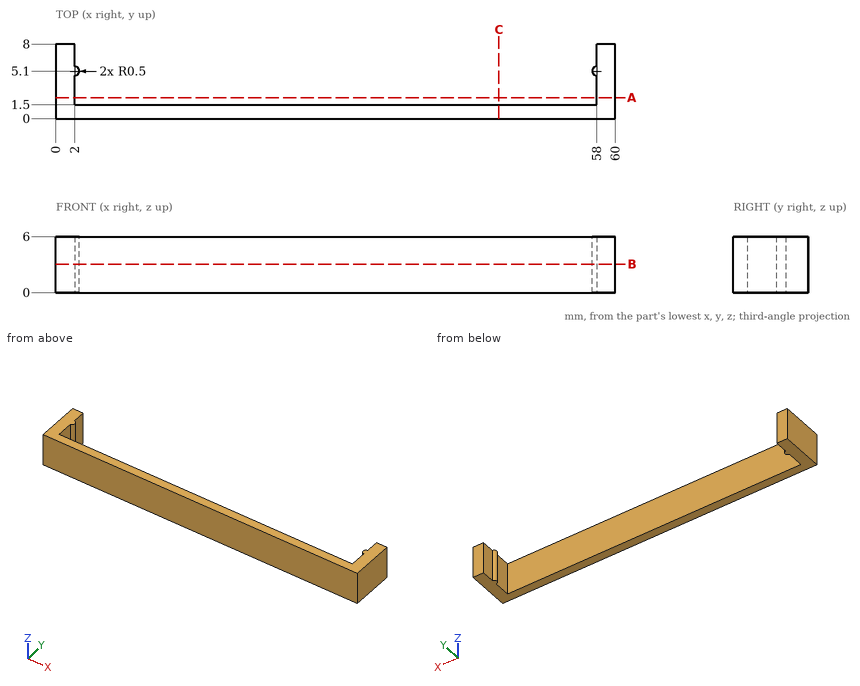
The figure shows three views and two pictorial views of one solid part (mm, origin at its lowest corner). Answer the questions. Round coordinates to 2 decimals unless told otherwise and drop trailing zeros. Order: outer loops, then holes, each group sorted by start corner. A loop starts at its lowest first (then second) coordinate and runs counter-clockwise, first axis right, second up.
Q1. A cutting plane is placed at C-C, the plane x = 47.5. Determine the outline of the cut face in (y, z).
Solution:
outline: (0, 0) - (1.5, 0) - (1.5, 6) - (0, 6) - close
Q2. Find the intervals of material crossed by line 1 along X through (y, z) = (4.25, 2.85); line 2 along Y through (x, z) = (12, 4.3); line 3 along X through (y, z) = (5.25, 5.25), in increasing order.
Solution:
line 1: x = 0 to 2, 58 to 60
line 2: y = 0 to 1.5
line 3: x = 0 to 2.48, 57.52 to 60
Q3. A cutting plane is placed at B-B, the plane z = 3.05. Determine the outline of the cut face in (x, y).
Solution:
outline: (0, 0) - (60, 0) - (60, 8) - (58, 8) - (58, 5.6) arc R0.5 ccw to (58, 4.6) - (58, 1.5) - (2, 1.5) - (2, 4.6) arc R0.5 ccw to (2, 5.6) - (2, 8) - (0, 8) - close
Q4. A cutting plane is placed at A-A, the plane y = 2.25. Determine the outline of the cut face in (x, z).
Solution:
outline: (0, 0) - (2, 0) - (2, 6) - (0, 6) - close; (58, 0) - (60, 0) - (60, 6) - (58, 6) - close
Q5. Given pin 1 Ø3 at (x, z) = (25.5, 2.5) entering from +Y; pin 2 Ø1 at (x, y) = (14.5, 2.5) entering from -Z, each flat-ended and moving along its own axis, determine where each tip first touches the part or whether it passes through.
Solution:
pin 1: stops at y = 1.5
pin 2: passes through
